Source: CAD feature listing. Evaluate the final solid. Frame: model axes, mm. A direction names the side the tool comes from. Round coordinates to 2 decimals unless told otherwise and drop trailing zeros. Loops run counter-clockwise (first coordinate to the right, second up) from the corner with the lowest first, then second, coordinate; pieces in that order, holes last. Notation, with made-up numbers: (20, 32) -> (54, 32) arc R18 ccw to (54, 54) -> close; hole circle Ø10 at (20.25, 41). An arc over 180 degrees is marked (long way). Write item = value, one per line.
from build123d import *

# Parameters (mm, degrees)
SKETCH1_W                = 150
SKETCH1_H                = 75
BOSS_EXTRUDE2_DEPTH      = 5
CUT_EXTRUDE9_DEPTH       = 6
CUT_EXTRUDE9_DEPTH_BACK  = 1
CUT_EXTRUDE10_DEPTH      = 1
CUT_EXTRUDE10_DEPTH_BACK = 6
FILLET3_R                = 8
FILLET4_R                = 8
FILLET5_R                = 8
FILLET6_R                = 8


with BuildPart() as part:
    # Sketch1 → Boss-Extrude2 (new body)
    with BuildSketch(Plane.XY):
        with Locations((75, 37.5)):
            Rectangle(SKETCH1_W, SKETCH1_H)
    extrude(amount=BOSS_EXTRUDE2_DEPTH)

    # Sketch2 → Cut-Extrude9 (cut, two sides)
    with BuildSketch(Plane.XY) as cut_extrude9_sk:
        with BuildLine():
            Line((56.039864316, 50), (56.039864316, 25))
            ThreePointArc((56.039864316, 25), (58.968796504, 17.928932188), (66.039864316, 15))
            Line((66.039864316, 15), (91.039864316, 15))
            ThreePointArc((91.039864316, 15), (98.110932128, 17.928932188), (101.039864316, 25))
            Line((101.039864316, 25), (101.039864316, 50))
            ThreePointArc((101.039864316, 50), (98.110932128, 57.071067812), (91.039864316, 60))
            Line((91.039864316, 60), (66.039864316, 60))
            ThreePointArc((66.039864316, 60), (58.968796504, 57.071067812), (56.039864316, 50))
        make_face()
        with BuildLine():
            Line((13, 0), (13, 40))
            ThreePointArc((13, 40), (20, 47), (27, 40))
            Line((27, 40), (27, 0))
            ThreePointArc((27, 0), (20, -7), (13, 0))
        make_face()
    extrude(amount=CUT_EXTRUDE9_DEPTH, mode=Mode.SUBTRACT)
    extrude(cut_extrude9_sk.sketch, amount=-CUT_EXTRUDE9_DEPTH_BACK, mode=Mode.SUBTRACT)

    # Sketch3 → Cut-Extrude10 (cut, two sides)
    with BuildSketch(Plane.XY.offset(5)) as cut_extrude10_sk:
        with BuildLine():
            Line((123, 397.371573611), (123, 75))
            Line((123, 75), (123, 35))
            ThreePointArc((123, 35), (130, 28), (137, 35))
            Line((137, 35), (137, 75))
            Line((137, 75), (137, 397.371573611))
            Line((137, 397.371573611), (137, 1042.114720832))
            Line((137, 1042.114720832), (123, 1042.114720832))
            Line((123, 1042.114720832), (123, 397.371573611))
        make_face()
    extrude(amount=CUT_EXTRUDE10_DEPTH, mode=Mode.SUBTRACT)
    extrude(cut_extrude10_sk.sketch, amount=-CUT_EXTRUDE10_DEPTH_BACK, mode=Mode.SUBTRACT)

    # Fillet3
    fillet3_edges = [part.edges().sort_by_distance(p)[0] for p in [
        (150, 75, 2.5),
    ]]
    fillet(fillet3_edges, radius=FILLET3_R)

    # Fillet4
    fillet4_edges = [part.edges().sort_by_distance(p)[0] for p in [
        (0, 0, 2.5),
    ]]
    fillet(fillet4_edges, radius=FILLET4_R)

    # Fillet5
    fillet5_edges = [part.edges().sort_by_distance(p)[0] for p in [
        (150, 0, 2.5),
    ]]
    fillet(fillet5_edges, radius=FILLET5_R)

    # Fillet6
    fillet6_edges = [part.edges().sort_by_distance(p)[0] for p in [
        (0, 75, 2.5),
    ]]
    fillet(fillet6_edges, radius=FILLET6_R)


solid = part.part
1. Section query A-A (z = 3.6). Return the cut outline in (x, y), then the cut area to 3 significant figures.
Evaluation:
outline = (0, 8) arc R8 ccw to (8, 0) -> (13, 0) -> (13, 40) arc R7 cw to (27, 40) -> (27, 0) -> (142, 0) arc R8 ccw to (150, 8) -> (150, 67) arc R8 ccw to (142, 75) -> (137, 75) -> (137, 35) arc R7 cw to (123, 35) -> (123, 75) -> (8, 75) arc R8 ccw to (0, 67) -> close; hole (56.04, 25) arc R10 ccw to (66.04, 15) -> (91.04, 15) arc R10 ccw to (101.04, 25) -> (101.04, 50) arc R10 ccw to (91.04, 60) -> (66.04, 60) arc R10 ccw to (56.04, 50) -> close
area = 7,980 mm²
2. Section query B-B (y = 65). Return the cut outline in (x, z), then the cut area to 3 significant figures.
Evaluation:
outline = (0, 0) -> (123, 0) -> (123, 5) -> (0, 5) -> close; (137, 0) -> (150, 0) -> (150, 5) -> (137, 5) -> close
area = 680 mm²
3. Set-up query: faces 1 (the face through (137, 55, 3)), 2 (the face through (10, 0, 2)), 3 (the face through (59, 57.1, 2.5)), 4 (the face through (27, 20, 2)). Return all of +Z, -Z, +X, -X, +Y, -Y with unobstructed straight access to the full face (end or side cutting, diameter ignored); none if empty.
Evaluation:
face_1 = +Z, -Z, +Y
face_2 = +Z, -Z, +X, -X, -Y
face_3 = +Z, -Z
face_4 = +Z, -Z, -Y
4. Mould query, pull axis X, two halves, no side actions, for faces 5 (the face through (123, 55, 3)), 6 (the face through (2.281, 2.406, 2.535)), 7 (the face through (147.594, 72.719, 2.535)), 8 (the face through (65, 75, 2)). Classes: released by +X, released by -X, zero draft, split by the parting line, or undercut.
Evaluation:
face_5 = undercut
face_6 = released by -X
face_7 = released by +X
face_8 = zero draft
5. Section query C-C (y = 18). Return the cut outline in (x, z).
Evaluation:
outline = (0, 0) -> (13, 0) -> (13, 5) -> (0, 5) -> close; (27, 0) -> (58.9, 0) -> (58.9, 5) -> (27, 5) -> close; (98.18, 0) -> (150, 0) -> (150, 5) -> (98.18, 5) -> close
6. Line query: probe 1 along X at (y, z) = (39.5, 4); probe 2 along X at (y, z) = (26.5, 2.7); probe 3 along X at (y, z) = (52, 0.9). Output: solid intervals per line, ascending. Write a range as from..to.
Evaluation:
probe_1 = 0..13, 27..56.04, 101.04..123, 137..150
probe_2 = 0..13, 27..56.04, 101.04..150
probe_3 = 0..56.24, 100.84..123, 137..150
7. Section query D-D (x = 130). Return the cut outline in (y, z), then the cut area to 3 significant figures.
Evaluation:
outline = (0, 0) -> (28, 0) -> (28, 5) -> (0, 5) -> close
area = 140 mm²
